Geometry check sheet. Reference: the model listing, model coordinates, mm. Face numbers are marked on the shaded views. A direction names the side the tool comes from. Coordinates: 2 decimals unless noted, no trailing zeros. Write each loop counter-clockwise with the first axis right and the second up, starting at its lowest first coordinate (ties: lowest second). Pieces come first, ordered by that corner, then holes. Notation, with made-up numbers: (73.25, 24) -> (82.25, 24) arc R5 cw to (82.25, 28) -> close; hole circle Ø3 at (-39, 65). An arc over 180 degrees is marked (long way). One line per question, with ' | ' between items.
```python
from build123d import *

# Parameters (mm, degrees)
ESQUISSE1_R             = 0.95
BOSS_EXTRU_1_DEPTH      = 5
ESQUISSE2_W             = 14
ESQUISSE2_H             = 13
ENL_V_MAT_EXTRU_1_DEPTH = 3
BOSS_EXTRU_3_DEPTH      = 3
CONG_4_R                = 0.5
CONG_5_R                = 0.2
SYM_TRIE2_START         = 5
SYM_TRIE2_DEPTH         = 3
CONG_6_R                = 2


# Read off the part's stored shape, not the designer's step: Symétrie2
with BuildPart() as part:
    # Esquisse1 → Boss.-Extru.1 (new body)
    with BuildSketch(Plane.XY):
        with BuildLine():
            Line((-11.5, -8), (-11.5, -10))
            ThreePointArc((-11.5, -10), (-10.767766953, -11.767766953), (-9, -12.5))
            Line((-9, -12.5), (9, -12.5))
            ThreePointArc((9, -12.5), (10.767766953, -11.767766953), (11.5, -10))
            Line((11.5, -10), (11.5, -8))
            ThreePointArc((11.5, -8), (8.44427191, 0), (11.5, 8))
            Line((11.5, 8), (11.5, 10))
            ThreePointArc((11.5, 10), (10.767766953, 11.767766953), (9, 12.5))
            Line((9, 12.5), (-9, 12.5))
            ThreePointArc((-9, 12.5), (-10.767766953, 11.767766953), (-11.5, 10))
            Line((-11.5, 10), (-11.5, 8))
            ThreePointArc((-11.5, 8), (-8.44427191, 0), (-11.5, -8))
        make_face()
        with Locations((-9, -10)):
            Circle(ESQUISSE1_R, mode=Mode.SUBTRACT)
        with Locations((9, -10)):
            Circle(ESQUISSE1_R, mode=Mode.SUBTRACT)
        with Locations((-9, 10)):
            Circle(ESQUISSE1_R, mode=Mode.SUBTRACT)
        with Locations((9, 10)):
            Circle(ESQUISSE1_R, mode=Mode.SUBTRACT)
    extrude(amount=BOSS_EXTRU_1_DEPTH)

    # Esquisse2 → Enlèv. mat.-Extru.1 (cut)
    with BuildSketch(Plane(origin=(0, 0, 0), x_dir=(-1, 0, 0), z_dir=(0, 0, -1))):
        Rectangle(ESQUISSE2_W, ESQUISSE2_H)
    extrude(amount=-ENL_V_MAT_EXTRU_1_DEPTH, mode=Mode.SUBTRACT)

    # Esquisse5 → Boss.-Extru.3 (add)
    with BuildSketch(Plane.XY.offset(5)):
        with BuildLine():
            Line((-10.253049234, 8), (-9.010874707, 8))
            ThreePointArc((-9.010874707, 8), (-6.5, 0), (-9.010874707, -8))
            Line((-9.010874707, -8), (-10.253049234, -8))
            ThreePointArc((-10.253049234, -8), (-7.5, 0), (-10.253049234, 8))
        make_face()
        with BuildLine():
            Line((-8.375702269, -8.5), (-7.140792906, -8.5))
            ThreePointArc((-7.140792906, -8.5), (-4.5, 0), (-7.140792906, 8.5))
            Line((-7.140792906, 8.5), (-8.375702269, 8.5))
            ThreePointArc((-8.375702269, 8.5), (-5.5, 0), (-8.375702269, -8.5))
        make_face()
        with BuildLine():
            Line((-6.891813234, 9.5), (-5.62560681, 9.5))
            ThreePointArc((-5.62560681, 9.5), (-2.5, 0), (-5.62560681, -9.5))
            Line((-5.62560681, -9.5), (-6.891813234, -9.5))
            ThreePointArc((-6.891813234, -9.5), (-3.5, 0), (-6.891813234, 9.5))
        make_face()
        with BuildLine():
            Line((-5.649367106, 10.75), (-4.330432809, 10.75))
            ThreePointArc((-4.330432809, 10.75), (-0.5, 0), (-4.330432809, -10.75))
            Line((-4.330432809, -10.75), (-5.649367106, -10.75))
            ThreePointArc((-5.649367106, -10.75), (-1.5, 0), (-5.649367106, 10.75))
        make_face()
        with BuildLine():
            Line((-4.458405421, 12), (-3.083592135, 12))
            ThreePointArc((-3.083592135, 12), (-1.34998742, 9.719934096), (0, 7.193747285))
            ThreePointArc((0, 7.193747285), (1.34998742, 9.719934096), (3.083592135, 12))
            Line((3.083592135, 12), (4.458405421, 12))
            ThreePointArc((4.458405421, 12), (1.691654483, 8.349425312), (0, 4.092676386))
            ThreePointArc((0, 4.092676386), (-1.691654483, 8.349425312), (-4.458405421, 12))
        make_face()
        with BuildLine():
            Line((-4.458405421, -12), (-3.083592135, -12))
            ThreePointArc((-3.083592135, -12), (-1.34998742, -9.719934096), (0, -7.193747285))
            ThreePointArc((0, -7.193747285), (1.34998742, -9.719934096), (3.083592135, -12))
            Line((3.083592135, -12), (4.458405421, -12))
            ThreePointArc((4.458405421, -12), (1.691654483, -8.349425312), (0, -4.092676386))
            ThreePointArc((0, -4.092676386), (-1.691654483, -8.349425312), (-4.458405421, -12))
        make_face()
    extrude(amount=BOSS_EXTRU_3_DEPTH)

    # Congé4
    cong_4_edges = [part.edges().sort_by_distance(p)[0] for p in [
        (4.458405421, 12, 6.5),
        (3.083592135, 12, 6.5),
        (0, 7.193747285, 6.5),
        (-3.083592135, 12, 6.5),
        (-4.458405421, 12, 6.5),
        (-4.330432809, 10.75, 6.5),
        (-5.649367106, 10.75, 6.5),
        (-5.62560681, 9.5, 6.5),
        (-6.891813234, 9.5, 6.5),
        (-7.140792906, 8.5, 6.5),
        (-8.375702269, 8.5, 6.5),
        (-9.010874707, 8, 6.5),
        (-10.253049234, 8, 6.5),
        (0, -7.193747285, 6.5),
        (4.458405421, -12, 6.5),
        (3.083592135, -12, 6.5),
        (-3.083592135, -12, 6.5),
        (-4.458405421, -12, 6.5),
        (-4.330432809, -10.75, 6.5),
        (-5.649367106, -10.75, 6.5),
        (-5.62560681, -9.5, 6.5),
        (-6.891813234, -9.5, 6.5),
        (-7.140792906, -8.5, 6.5),
        (-8.375702269, -8.5, 6.5),
        (-9.010874707, -8, 6.5),
        (-10.253049234, -8, 6.5),
    ]]
    fillet(cong_4_edges, radius=CONG_4_R - 0.0001)  # a hair under: the kernel refuses the full size

    # Congé5
    cong_5_edges = [part.edges().sort_by_distance(p)[0] for p in [
        (0, 4.092676386, 6.5),
        (0, -4.092676386, 6.5),
    ]]
    fillet(cong_5_edges, radius=CONG_5_R)

    # Symétrie2 outline → Symétrie2 (add)
    with BuildSketch(Plane.XY.offset(SYM_TRIE2_START)):
        with BuildLine():
            ThreePointArc((9.27502784, -8), (9.715986392, -7.73570226), (9.690767549, -7.222222222))
            ThreePointArc((9.690767549, -7.222222222), (7.5, 0), (9.690767549, 7.222222222))
            ThreePointArc((9.690767549, 7.222222222), (9.715986392, 7.73570226), (9.27502784, 8))
            ThreePointArc((9.27502784, 8), (9.039325579, 7.940958552), (8.85928813, 7.777777778))
            ThreePointArc((8.85928813, 7.777777778), (6.5, 0), (8.85928813, -7.777777778))
            ThreePointArc((8.85928813, -7.777777778), (9.039325579, -7.940958552), (9.27502784, -8))
        make_face()
        with BuildLine():
            ThreePointArc((7.406613378, -8.5), (7.847028542, -8.236716038), (7.823626709, -7.724137931))
            ThreePointArc((7.823626709, -7.724137931), (5.5, 0), (7.823626709, 7.724137931))
            ThreePointArc((7.823626709, 7.724137931), (7.847028542, 8.236716038), (7.406613378, 8.5))
            ThreePointArc((7.406613378, 8.5), (7.169897339, 8.440415165), (6.989600046, 8.275862069))
            ThreePointArc((6.989600046, 8.275862069), (4.5, 0), (6.989600046, -8.275862069))
            ThreePointArc((6.989600046, -8.275862069), (7.169897339, -8.440415165), (7.406613378, -8.5))
        make_face()
        with BuildLine():
            ThreePointArc((5.880570536, -9.5), (6.32507098, -9.228952735), (6.287648906, -8.709677419))
            ThreePointArc((6.287648906, -8.709677419), (3.5, 0), (6.287648906, 8.709677419))
            ThreePointArc((6.287648906, 8.709677419), (6.32507098, 9.228952735), (5.880570536, 9.5))
            ThreePointArc((5.880570536, 9.5), (5.651617801, 9.444500445), (5.473492166, 9.290322581))
            ThreePointArc((5.473492166, 9.290322581), (2.5, 0), (5.473492166, -9.290322581))
            ThreePointArc((5.473492166, -9.290322581), (5.651617801, -9.444500445), (5.880570536, -9.5))
        make_face()
        with BuildLine():
            ThreePointArc((4.569899459, -10.75), (5.020067778, -10.46759707), (4.961720688, -9.939393939))
            ThreePointArc((4.961720688, -9.939393939), (1.5, 0), (4.961720688, 9.939393939))
            ThreePointArc((4.961720688, 9.939393939), (5.020067778, 10.46759707), (4.569899459, 10.75))
            ThreePointArc((4.569899459, 10.75), (4.352302389, 10.700168319), (4.17807823, 10.560606061))
            ThreePointArc((4.17807823, 10.560606061), (0.5, 0), (4.17807823, -10.560606061))
            ThreePointArc((4.17807823, -10.560606061), (4.352302389, -10.700168319), (4.569899459, -10.75))
        make_face()
    extrude(amount=SYM_TRIE2_DEPTH)

    # Congé6
    cong_6_edges = [part.edges().sort_by_distance(p)[0] for p in [
        (11.5, 8, 2.5),
        (11.5, -8, 2.5),
        (-11.5, -8, 2.5),
        (-11.5, 8, 2.5),
    ]]
    fillet(cong_6_edges, radius=CONG_6_R)


solid = part.part
```
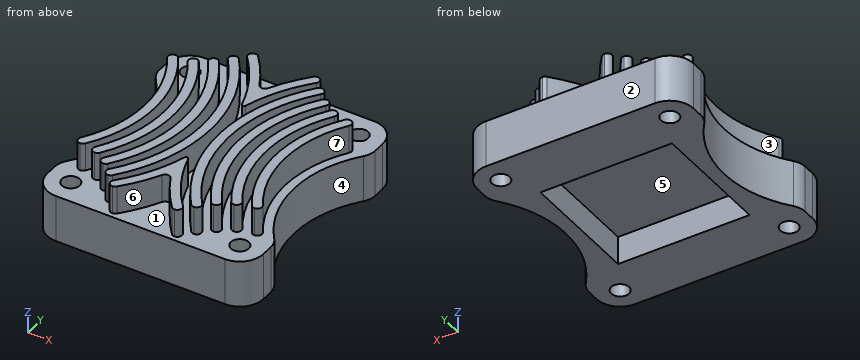
(1) Draft check along X on the marked faces 1, 2, 3 and 4. Enter one of: pulls with the +X half, pulls with the -X half, needs draft (parallel to the pull), parting line crosses it, or undercut.
Answers below:
face 1: undercut | face 2: needs draft | face 3: pulls with the -X half | face 4: pulls with the +X half
(2) Material ranges on line 1 (Y direction, x = 6.75, z = 2); line 2 (X direction, y = -3.75, z = 2); line 3 (X direction, y = 10.5, z = 3.75), recorded low to high.
Answers below:
line 1: y = -12.5 to -6.5, 6.5 to 12.5 | line 2: x = -9.05 to -7, 7 to 9.05 | line 3: x = -11.45 to -9.81, -8.19 to 8.19, 9.81 to 11.45
(3) Cross-section at A-A (z = 2). Record the cut outline in (x, y).
Answers below:
outline: (-11.5, -10) arc R2.5 ccw to (-9, -12.5) -> (9, -12.5) arc R2.5 ccw to (11.5, -10) -> (11.5, -8.73) arc R2 ccw to (11.06, -7.48) arc R12 cw to (11.06, 7.48) arc R2 ccw to (11.5, 8.73) -> (11.5, 10) arc R2.5 ccw to (9, 12.5) -> (-9, 12.5) arc R2.5 ccw to (-11.5, 10) -> (-11.5, 8.73) arc R2 ccw to (-11.06, 7.48) arc R12 cw to (-11.06, -7.48) arc R2 ccw to (-11.5, -8.73) -> close; hole circle Ø1.9 at (-9, -10); hole circle Ø1.9 at (-9, 10); hole (-7, -6.5) -> (7, -6.5) -> (7, 6.5) -> (-7, 6.5) -> close; hole circle Ø1.9 at (9, -10); hole circle Ø1.9 at (9, 10)
(4) Cross-section at B-B (z = 4). Record the cut outline in (x, y).
Answers below:
outline: (-11.5, -10) arc R2.5 ccw to (-9, -12.5) -> (9, -12.5) arc R2.5 ccw to (11.5, -10) -> (11.5, -8.73) arc R2 ccw to (11.06, -7.48) arc R12 cw to (11.06, 7.48) arc R2 ccw to (11.5, 8.73) -> (11.5, 10) arc R2.5 ccw to (9, 12.5) -> (-9, 12.5) arc R2.5 ccw to (-11.5, 10) -> (-11.5, 8.73) arc R2 ccw to (-11.06, 7.48) arc R12 cw to (-11.06, -7.48) arc R2 ccw to (-11.5, -8.73) -> close; hole circle Ø1.9 at (-9, -10); hole circle Ø1.9 at (-9, 10); hole circle Ø1.9 at (9, -10); hole circle Ø1.9 at (9, 10)
(5) Depth check by flat-ended pin: P1, Ø1.7, axis at x = -9, y = 10, coming from the -Z side; P2, Ø4, axis at x = 0.5, y = 3, coming from the -Z side; P3, Ø2, axis at y = -7.5, z = 3, coming from the +X side; P4, Ø1, axis at y = -4.5, z = 4.5, coming from the +X side. Enter the tip coordinate at first touch or a pass-through.
Answers below:
P1: passes through | P2: stops at z = 3 | P3: stops at x = 11.49 | P4: stops at x = 9.54
(6) Tool access check on the marked faces 5, 6 and 7. Record the directions out of +Z, -Z, +X, -X, +Y, -Y that give a thin tool (end or side, any length) a straight path to the whole face; none if there is none.
Answers below:
face 5: -Z | face 6: +Z, -Y | face 7: +Z, +X
